from build123d import *

# Parameters (mm, degrees)
SKETCH1_W                = 74
SKETCH1_H                = 74
SKETCH1_W_2              = 54
SKETCH1_H_2              = 54
BOSS_EXTRUDE1_DEPTH      = 3
M3_CLEARANCE_HOLE1_D     = 3.2
M3_CLEARANCE_HOLE1_DEPTH = 4.5
M3_CLEARANCE_HOLE1_TIP   = 0.96137699
FILLET1_R                = 5


with BuildPart() as part:
    # Sketch1 → Boss-Extrude1 (new body)
    with BuildSketch(Plane(origin=(0, 0, 0), x_dir=(1, 0, 0), z_dir=(0, 1, 0))):
        Rectangle(SKETCH1_W, SKETCH1_H)
        Rectangle(SKETCH1_W_2, SKETCH1_H_2, mode=Mode.SUBTRACT)
    extrude(amount=BOSS_EXTRUDE1_DEPTH)

    # M3 Clearance Hole1
    with Locations(Plane(origin=(-30.5, 3, -32.5), x_dir=(0, 0, 1), z_dir=(0, 1, 0))):
        with Locations((0, 0), (0, 61), (65, 61), (65, 0)):
            Hole(M3_CLEARANCE_HOLE1_D / 2, depth=M3_CLEARANCE_HOLE1_DEPTH)
            with Locations((0, 0, -(M3_CLEARANCE_HOLE1_DEPTH + M3_CLEARANCE_HOLE1_TIP / 2))):  # 118° drill point
                Cone(0, M3_CLEARANCE_HOLE1_D / 2, M3_CLEARANCE_HOLE1_TIP, mode=Mode.SUBTRACT)

    # Fillet1
    fillet1_edges = [part.edges().sort_by_distance(p)[0] for p in [
        (37, 1.5, 37),
        (-37, 1.5, 37),
        (-37, 1.5, -37),
        (37, 1.5, -37),
    ]]
    fillet(fillet1_edges, radius=FILLET1_R)


solid = part.part
Part model, mm, in its own coordinate system. A direction names the side the tool comes from. Round coordinates to 2 decimals unless told otherwise and drop trailing zeros. Order: outer loops, then holes, each group sorted by start corner. A loop starts at its lowest first (then second) coordinate and runs counter-clockwise, first axis right, second up. Notation, with made-up numbers: (-12, 33) -> (37, 33) arc R28 cw to (37, 67) -> close; hole circle Ø8 at (70.25, 86.5). An arc over 180 degrees is marked (long way). Put each result on its own line as item: value.
Q1. Band-saw the part on D-D (z = 14.5). Give the cut face in (x, y).
From the geometry:
outline: (-37, 0) -> (-27, 0) -> (-27, 3) -> (-37, 3) -> close; (27, 0) -> (37, 0) -> (37, 3) -> (27, 3) -> close
Q2. Band-saw the part on B-B (y = 0.75). Give the cut face in (x, z).
From the geometry:
outline: (-37, -32) arc R5 ccw to (-32, -37) -> (32, -37) arc R5 ccw to (37, -32) -> (37, 32) arc R5 ccw to (32, 37) -> (-32, 37) arc R5 ccw to (-37, 32) -> close; hole circle Ø3.2 at (-30.5, -32.5); hole circle Ø3.2 at (-30.5, 32.5); hole (-27, -27) -> (27, -27) -> (27, 27) -> (-27, 27) -> close; hole circle Ø3.2 at (30.5, -32.5); hole circle Ø3.2 at (30.5, 32.5)
Q3. Band-saw the part on A-A (x = 30.5). Give the cut face in (y, z).
From the geometry:
outline: (0, -37) -> (3, -37) -> (3, -34.1) -> (0, -34.1) -> close; (0, -30.9) -> (3, -30.9) -> (3, 30.9) -> (0, 30.9) -> close; (0, 34.1) -> (3, 34.1) -> (3, 37) -> (0, 37) -> close
Q4. Band-saw the part on C-C (x = 21). Give the cut face in (y, z).
From the geometry:
outline: (0, -37) -> (3, -37) -> (3, -27) -> (0, -27) -> close; (0, 27) -> (3, 27) -> (3, 37) -> (0, 37) -> close
Q5. Wall check: line 1 (Z direction, x = 21.5, y = 1.3); line 2 (Z direction, x = -31, y = 0.4). Give the ranges that are in metal, low to high. Write a range as [from, to].
From the geometry:
line 1: z = [-37, -27], [27, 37]
line 2: z = [-37, -34.02], [-30.98, 30.98], [34.02, 37]
Q6. Tool access for faces 4 (the face through (-33, 3, -1)), 5 (the face through (0, 1, 27)): list every direction of +Z, -Z, +X, -X, +Y, -Y with a clear straight run to the whole face (end or side of a thin tool).
From the geometry:
face 4: +Z, -Z, +X, -X, +Y
face 5: +Y, -Y
Q7. Pull direction Z, two halves, no side cores. Call faces 1 (the face through (-37, 1, 0)), 2 (the face through (30.57, 1.48, 34.1)), 3 (the face through (-36, 2, 35)): pulls with the +Z half, pulls with the -Z half, needs draft (parallel to the pull), parting line crosses it, or undercut.
From the geometry:
face 1: needs draft
face 2: undercut
face 3: pulls with the +Z half
